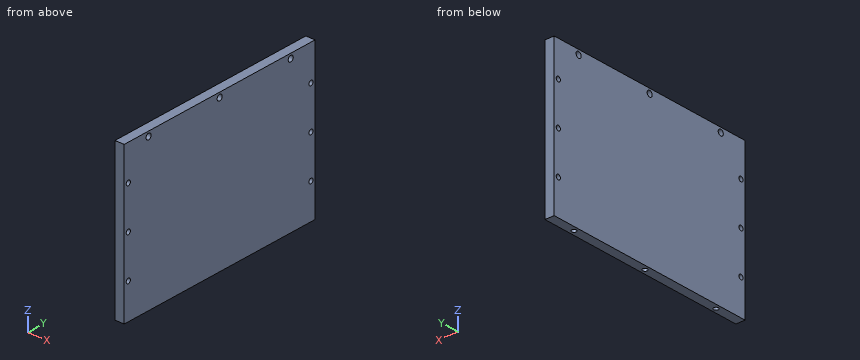
from build123d import *

# Parameters (mm, degrees)
SKETCH_1_R               = 1.25
EXTRUDE_1_DEPTH          = 4
HOLE_WIZARD_M2_5_1_D     = 2.05
HOLE_WIZARD_M2_5_2_D     = 2.05
HOLE_WIZARD_M2_5_2_DEPTH = 7.25
HOLE_WIZARD_M2_5_2_TIP   = 0.615882135


with BuildPart() as part:
    # 草图1 → 凸台-拉伸1 (new body)
    with BuildSketch(Plane(origin=(0, 0, 0), x_dir=(0, 0, -1), z_dir=(1, 0, 0))):
        Polygon((0, 0), (0, 47), (66, 47), (66, -47), (0, -47), align=None)
        with Locations((2, 0)):
            Circle(SKETCH_1_R, mode=Mode.SUBTRACT)
        with Locations((2, 35)):
            Circle(SKETCH_1_R, mode=Mode.SUBTRACT)
        with Locations((2, -35)):
            Circle(SKETCH_1_R, mode=Mode.SUBTRACT)
    extrude(amount=EXTRUDE_1_DEPTH)

    # M2.5 螺纹孔1 (through all)
    with Locations(Plane(origin=(4, 0, 0), x_dir=(0, 0, -1), z_dir=(1, 0, 0))):
        with Locations((15, 45), (51, 45), (15, -45), (51, -45), (33, -45), (33, 45)):
            Hole(HOLE_WIZARD_M2_5_1_D / 2)

    # M2.5 螺纹孔2
    with Locations(Plane(origin=(0, 0, -66), x_dir=(-1, 0, 0), z_dir=(0, 0, -1))):
        with Locations((-2, 35), (-2, 0), (-2, -35)):
            Hole(HOLE_WIZARD_M2_5_2_D / 2, depth=HOLE_WIZARD_M2_5_2_DEPTH)
            with Locations((0, 0, -(HOLE_WIZARD_M2_5_2_DEPTH + HOLE_WIZARD_M2_5_2_TIP / 2))):  # 118° drill point
                Cone(0, HOLE_WIZARD_M2_5_2_D / 2, HOLE_WIZARD_M2_5_2_TIP, mode=Mode.SUBTRACT)


solid = part.part
Work out the finished part from the listing and answer in its coordinate system (mm). Coordinates: 2 decimals unless noted, no trailing zeros. Write each loop counter-clockwise with the first axis right and the second up, starting at its lowest first coordinate (ties: lowest second). Pieces come first, ordered by that corner, then holes.
1. Consider line 1 along Y through (x, z) = (1.7, -2); line 2 along Y through (x, z) = (1, -15) (3 decimals); line 3 along X through (y, z) = (0, -62) (3 decimals). Determine where each line is inside the solid, lowest interval first.
Results list:
line 1: y = -47 to -36.25, -33.75 to -1.25, 1.25 to 33.75, 36.25 to 47
line 2: y = -47 to -46.025, -43.975 to 43.975, 46.025 to 47
line 3: x = 0 to 0.975, 3.025 to 4
2. The part is cut by section A-A, the plane z = -51. Write down the section's boundary in (x, y) (3 decimals), and give its area (3 significant figures).
Results list:
outline: (0, -47) - (4, -47) - (4, -46.025) - (0, -46.025) - close; (0, -43.975) - (4, -43.975) - (4, 43.975) - (0, 43.975) - close; (0, 46.025) - (4, 46.025) - (4, 47) - (0, 47) - close
area: 360 mm2
3. Flat-ended cylindrical pins translate along their axes: pin 1 (3.5 mm diameter, centred on y = -45, z = -33, fed in from -X); pin 2 (1.8 mm diameter, centred on y = -45, z = -15, fed in from +X). Find the tip coordinate at first contact, or state that the pin passes through.
Results list:
pin 1: stops at x = 0
pin 2: passes through
4. The part is cut by section B-B, the plane y = 45. Write down the section's boundary in (x, z) (3 decimals).
Results list:
outline: (0, -66) - (4, -66) - (4, -52.025) - (0, -52.025) - close; (0, -49.975) - (4, -49.975) - (4, -34.025) - (0, -34.025) - close; (0, -31.975) - (4, -31.975) - (4, -16.025) - (0, -16.025) - close; (0, -13.975) - (4, -13.975) - (4, 0) - (0, 0) - close
